Autodesk Inventor part; units mm, degrees
ref_plane "YZ Plane" through (0, 0, 0) normal (1, 0, 0) x (0, 1, 0)
ref_plane "XZ Plane" through (0, 0, 0) normal (0, 1, 0) x (-1, 0, 0)
ref_plane "XY Plane" through (0, 0, 0) normal (0, 0, 1) x (1, 0, 0)
sketch "Sketch1" plane through (0, 0, 0) normal (0, 1, 0) x (-1, 0, 0)
  circle A0 centre (28, -4.85) radius 1.6
  line L0 (28, -8.0832) -> (25.2, -6.4666)
  line L1 (25.2, -6.4666) -> (25.2, -3.2334)
  line L2 (25.2, -3.2334) -> (28, -1.6168)
  line L3 (28, -1.6168) -> (30.8, -3.2334)
  line L4 (30.8, -3.2334) -> (30.8, -6.4666)
  line L5 (30.8, -6.4666) -> (28, -8.0832)
  line L6 (-16, -20.0067) -> (-16, -32.5067)
  line L7 (37, -52.1) -> (37, 0)
  line L8 (-16, -32.5067) -> (-19, -32.5067)
  line L9 (-16, -20.0067) -> (-19, -20.0067)
  line L10 (-12.8, -32.5067) -> (-12.8, -20.0067)
  line L11 (-12.8, -20.0067) -> (-9.8, -20.0067)
  line L12 (-9.8, -20.0067) -> (-9.8, -32.5067)
  line L13 (-9.8, -32.5067) -> (-12.8, -32.5067)
  line L14 (33.8, -32.3) -> (30.8, -32.3)
  line L15 (30.8, -32.3) -> (30.8, -19.8)
  line L16 (30.8, -19.8) -> (33.8, -19.8)
  line L17 (33.8, -19.8) -> (33.8, -32.3)
  line L18 (27.6, -32.3) -> (27.6, -19.8)
  line L19 (27.6, -19.8) -> (24.6, -19.8)
  line L20 (24.6, -19.8) -> (24.6, -32.3)
  line L21 (24.6, -32.3) -> (27.6, -32.3)
  line L22 (-19, -20.0067) -> (-19, -32.5067)
  line L23 (37, 0) -> (-19, 0)
  line L24 (-19, 0) -> (-19, -52.1)
  line L25 (-19, -52.1) -> (37, -52.1)
  circle A1 centre (-10, -4.85) radius 1.6
  line L26 (-10, -8.0832) -> (-12.8, -6.4666)
  line L27 (-12.8, -6.4666) -> (-12.8, -3.2334)
  line L28 (-12.8, -3.2334) -> (-10, -1.6168)
  line L29 (-10, -1.6168) -> (-7.2, -3.2334)
  line L30 (-7.2, -3.2334) -> (-7.2, -6.4666)
  line L31 (-7.2, -6.4666) -> (-10, -8.0832)
  circle A2 centre (-10, -45.05) radius 1.6
  line L32 (-10, -48.2832) -> (-12.8, -46.6666)
  line L33 (-7.2, -46.6666) -> (-10, -48.2832)
  line L34 (-7.2, -43.4334) -> (-7.2, -46.6666)
  line L35 (-12.8, -46.6666) -> (-12.8, -43.4334)
  line L36 (-10, -41.8168) -> (-7.2, -43.4334)
  line L37 (-12.8, -43.4334) -> (-10, -41.8168)
  line L38 (30.8, -46.6666) -> (28, -48.2832)
  line L39 (28, -48.2832) -> (25.2, -46.6666)
  circle A3 centre (28, -45.05) radius 1.6
  line L40 (30.8, -43.4334) -> (30.8, -46.6666)
  line L41 (28, -41.8168) -> (30.8, -43.4334)
  line L42 (25.2, -46.6666) -> (25.2, -43.4334)
  line L43 (25.2, -43.4334) -> (28, -41.8168)
  line L44 (-2.45, -26.1) -> (17.25, -26.1)
  line L45 (17.25, -26.1) -> (17.25, -52.1)
  line L46 (17.25, -52.1) -> (-2.45, -52.1)
  line L47 (-2.45, -52.1) -> (-2.45, -26.1)
  point P0 (-17.5, -20.0067)
  point P1 (26.1, -19.8)
  point P2 (-11.3, -20.0067)
  point P3 (32.3, -32.3)
  point P4 (30.8, -4.85)
  point P5 (-7.2, -4.85)
  point P6 (-7.2, -45.05)
  point P7 (30.8, -45.05)
  point P8 (-12.8, -45.05)
  dimension "d2" = 3.2
  dimension "d5" = 5.6
  dimension "d63" = 3.2
  dimension "d64" = 3
  dimension "d65" = 3
  dimension "d67" = 12.5
  dimension "d69" = 3.2
  dimension "d70" = 3.2
  dimension "d71" = 12.5
  dimension "d121" = 3.2
  dimension "d122" = 5.6
  dimension "d123" = 4.85
  dimension "d124" = 4.85
  dimension "d126" = 6.2
  dimension "d128" = 3.2
  dimension "d129" = 5.6
  dimension "d130" = 3.2
  dimension "d131" = 5.6
  dimension "d133" = 56
  dimension "d137" = 7.05
  dimension "d138" = 52.1
  dimension "d139" = 40.2
  dimension "d140" = 7.05
  dimension "d141" = 6.2
  dimension "d143" = 19.7
  dimension "d144" = 26
  dimension "d147" = 0
  dimension "d148" = 34.4
  dimension "d149" = 7.35
  dimension "d150" = 16.55
  dimension "d161" = 6.2
  dimension "d163" = 6.2
extrude "Extrusão6" add sketch "Sketch1" against normal blind 4 contours A0 | L0 L1 L2 L3 L4 L5 | L9 L24 L23 L7 L25 L45 L44 L47 L8 L6 | L6 L8 L22 L9 | L47 L44 L45 L25 | L10 L11 L12 L13 | L14 L15 L16 L17 | L21 L20 L19 L18 | A1 | L26 L27 L28 L29 L30 L31 | A2 | L32 L35 L37 L36 L34 L33 | L38 L39 L42 L43 L41 L40 | A3
extrude "Extrusão7" add sketch "Sketch1" along normal blind 30 contours L6 L8 L22 L9 | L10 L11 L12 L13 | L14 L15 L16 L17 | L21 L20 L19 L18
fillet "Arredondamento5" radius 6.25 8 edges at (17.5, 30, -20.0067) (17.5, 30, -32.5067) (11.3, 30, -32.5067) (11.3, 30, -20.0067) (-26.1, 30, -19.8) (-26.1, 30, -32.3) (-32.3, 30, -32.3) (-32.3, 30, -19.8)
fillet "Arredondamento7" radius 8.5 8 edges at (17.5, 0, -32.5067) (11.3, 0, -32.5067) (-26.1, 0, -32.3) (-32.3, 0, -32.3) (-32.3, 0, -19.8) (-26.1, 0, -19.8) (11.3, 0, -20.0067) (17.5, 0, -20.0067)
extrude "Extrusão13" cut sketch "Sketch1" against normal blind 10 contours L47 L44 L45 L25
extrude "Extrusão14" cut sketch "Sketch1" against normal blind 10 contours A0 | A1 | A2 | A3
extrude "Extrusão15" cut sketch "Sketch1" against normal blind 2 contours L0 L1 L2 L3 L4 L5 | A1 | L26 L27 L28 L29 L30 L31 | L32 L35 L37 L36 L34 L33 | L38 L39 L42 L43 L41 L40 | A3
sketch "Esboço4" plane through (-33.8, 23.75, -26.05) normal (-1, 0, 0) x (0, 0, 1)
  circle A0 centre (0, 0) radius 1.65
  point P0 (26.05, -23.75)
  dimension "d158" = 3.3
extrude "Extrusão16" cut sketch "Esboço4" against normal blind 100
properties part number "encaixeDuplo3"
The listing builds one solid part. Answer for the finished solid, in the listing's coordinates (mm). A direction names the side the tool comes from. Round coordinates to 2 decimals unless told otherwise and drop trailing zeros. Order: outer loops, then holes, each group sorted by start corner. A loop starts at its lowest first (then second) coordinate and runs counter-clockwise, first axis right, second up. Notation, with made-up numbers: (-38.5, 25.5) -> (-32.5, 25.5) arc R28 ccw to (-32.5, 49.5) -> close; hole circle Ø8 at (80.5, 43.5). An arc over 180 degrees is marked (long way). Answer as CSV lines item,"result". Start each with the question number.
(1) The part is cut by section C-C (z = -28.5). Determine the outline of the cut face in (x, y).
(2) A tool of negligible diameter and unlimited length cuts with its end or side. For faces 1 (the face through (-26.58, -0.986, -42.636)), 2 (the face through (17.52, 28.22, -21.89)), 3 (the face through (-7, -2, -26.1)), 4 (the face through (17, 16, -32.507)), 5 (the face through (-32.28, 28.12, -30.52)), from which of +Z, -Z, +X, -X, +Y, -Y can it reach the whole face along a straight path? Write none if from no direction.
(3) For a pull along Y with two mould halves and no side action, classify faces 6 (the face through (11.279, 24.865, -27.266)), 7 (the face through (-26.08, 2.42, -17.24)), 8 (the face through (-25.2, -1, -45)) as +Y half, -Y half, draft (parallel to the pull), parting line (faces both ways), or undercut.
(4) Find the intervals of material crossed by probe 1 along X at (y, z) = (18.5, -28.5); probe 2 along Z at (x, y) = (10, -3); probe 3 along Y at (x, z) = (18.1, -26.05), in increasing order. Write a range as from..to.
(5) The part is cut by section A-A (z = -45.05). Determine the outline of the cut face in (x, y).
(6) Flat-ended cylindrical pins translate along their axes: pin 1 Ø0.9 at (x, y) = (-32, 16) entering from -Z; pin 2 Ø10 at (x, y) = (-10.5, 8.5) entering from +Z; pin 3 Ø3.5 at (x, y) = (11.5, 13) entering from -Z; pin 4 Ø2 at (x, y) = (11, 10.5) entering from +Z. Find the tip coordinate at first contact, or state that the pin passes through.
(7) The part is cut by section D-D (x = -18). Determine the outline of the cut face in (y, z), then the cut area to 3 significant figures.
(8) The part is cut by section B-B (y = 27.5). Determine the outline of the cut face in (x, z).
Evaluation:
1,outline,"(-37, -4) -> (-17.25, -4) -> (-17.25, 0) -> (-24.6, 0) -> (-24.6, 29.5) -> (-27.6, 29.5) -> (-27.6, 0) -> (-30.8, 0) -> (-30.8, 29.5) -> (-33.8, 29.5) -> (-33.8, 0) -> (-37, 0) -> close; (2.45, -4) -> (19, -4) -> (19, 29.58) -> (16, 29.58) -> (16, 0) -> (12.8, 0) -> (12.8, 29.58) -> (9.8, 29.58) -> (9.8, 0) -> (2.45, 0) -> close"
2,face 1,"+Y"
2,face 2,"+Z, +X, +Y"
2,face 3,"-Z, +Y, -Y"
2,face 4,"-Z, +X, -X, +Y"
2,face 5,"-Z, -X, +Y"
3,face 6,"undercut"
3,face 7,"+Y half"
3,face 8,"draft"
4,probe 1,"-33.8..-30.8, -27.6..-24.6, 9.8..12.8, 16..19"
4,probe 2,"-52.1..-46.65, -43.45..-6.45, -3.25..0"
4,probe 3,"-4..22.1, 25.4..30"
5,outline,"(-37, -4) -> (-29.6, -4) -> (-29.6, -2) -> (-30.8, -2) -> (-30.8, 0) -> (-37, 0) -> close; (-26.4, -4) -> (-17.25, -4) -> (-17.25, 0) -> (-25.2, 0) -> (-25.2, -2) -> (-26.4, -2) -> close; (2.45, -4) -> (8.4, -4) -> (8.4, -2) -> (7.2, -2) -> (7.2, 0) -> (2.45, 0) -> close; (11.6, -4) -> (19, -4) -> (19, 0) -> (12.8, 0) -> (12.8, -2) -> (11.6, -2) -> close"
6,pin 1,"z = -32.3"
6,pin 2,"through"
6,pin 3,"z = -32.51"
6,pin 4,"z = -20.01"
7,outline,"(-4, -52.1) -> (0, -52.1) -> (0, 0) -> (-4, 0) -> close"
7,area,"208 mm²"
8,outline,"(-33.8, -31.05) -> (-30.8, -31.05) -> (-30.8, -21.05) -> (-33.8, -21.05) -> close; (-27.6, -31.05) -> (-24.6, -31.05) -> (-24.6, -21.05) -> (-27.6, -21.05) -> close; (9.8, -31.26) -> (12.8, -31.26) -> (12.8, -21.26) -> (9.8, -21.26) -> close; (16, -31.26) -> (19, -31.26) -> (19, -21.26) -> (16, -21.26) -> close"
